Part print with two shaded views. Sizes in mm from the minimum x, y, z corner. Give positions to 0.01 mm unless a question says otherwise; leave off trailing zeros. Write each loop counter-clockwise with the first axis right and the second up, starting at its lowest first coordinate (ties: lowest second). Pieces come first, ordered by that corner, then holes. Notation, with made-up numbers: (-1.75, 65.25) - (29.25, 65.25) arc R32 cw to (29.25, 96.25) - close; hole circle Ø4 at (-13, -25). An arc over 180 degrees is marked (long way). One line per item, written item: value. Start each with the question number.
(1) Probe L1, parallel to Y at x = 3.5, z = 1 (1 decimal); L2, parallel to X at y = 2.5, z = 2.75 (1 decimal); L3, parallel to X at y = 1.25, z = 2.55 (1 decimal). List the from-to ranges inside material, lowest first.
(2) Cut at C-C, the plane y = 4.5. List the corners of the cut face in (x, z) (1 decimal).
(3) Cut at D-D, the plane x = 0.5. List the corners of the cut face in (y, z).
(4) Cut at B-B, the plane z = 0.8. List the corners of the cut face in (x, y).
(5) Mould opens along Y. For the marked faces 1, 2 and 3 say: pulls with the +Y half, pulls with the -Y half, needs draft (parallel to the pull), parting line crosses it, or undercut.
(6) Drop a flat-ended pin along its axis: P1, Ø1.5, axis at x = 9, y = 2, coming from the -Z side. Give the stop position or say it passes through.
(7) Cut at A-A, the plane x = 5.5. List the corners of the cut face in (y, z).
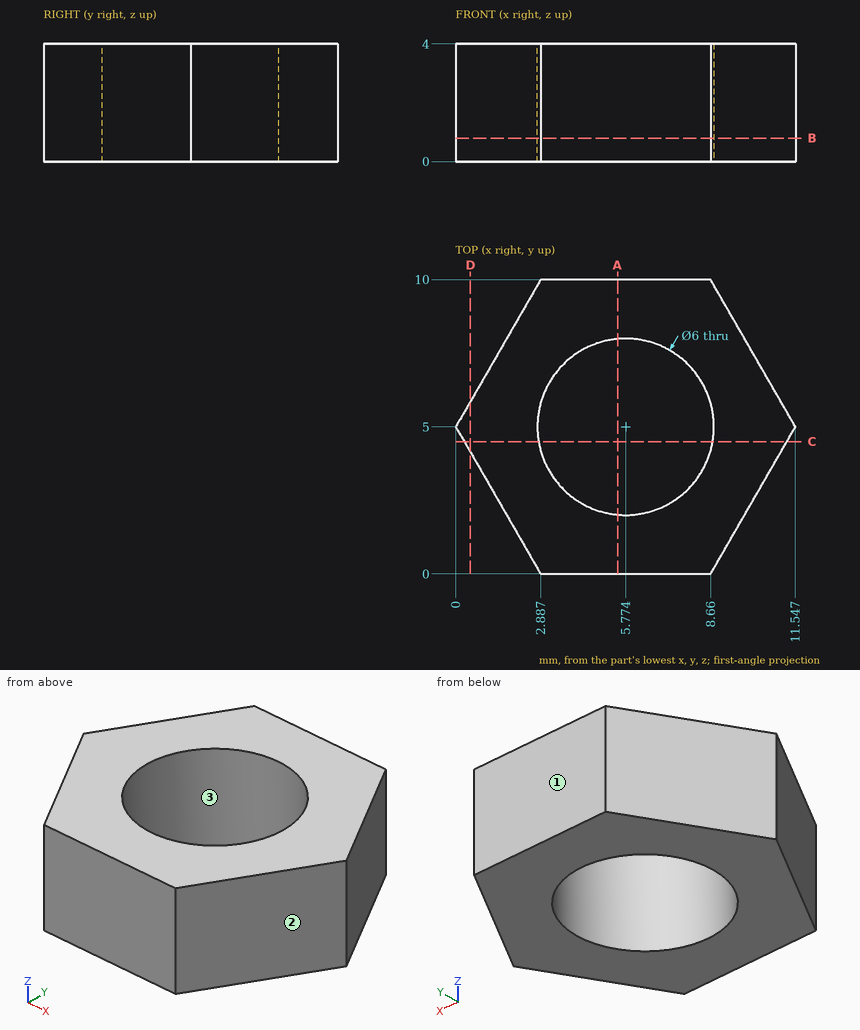
Answers follow:
1. L1: y = 0 to 3, 7 to 10
1. L2: x = 1.4 to 4.1, 7.4 to 10.1
1. L3: x = 2.2 to 9.4
2. outline: (0.3, 0) - (2.8, 0) - (2.8, 4) - (0.3, 4) - close; (8.7, 0) - (11.3, 0) - (11.3, 4) - (8.7, 4) - close
3. outline: (4.13, 0) - (5.87, 0) - (5.87, 4) - (4.13, 4) - close
4. outline: (0, 5) - (2.89, 0) - (8.66, 0) - (11.55, 5) - (8.66, 10) - (2.89, 10) - close; hole circle Ø6 at (5.77, 5)
5. face 1: pulls with the +Y half
5. face 2: pulls with the -Y half
5. face 3: undercut
6. P1: stops at z = 0
7. outline: (0, 0) - (2.01, 0) - (2.01, 4) - (0, 4) - close; (7.99, 0) - (10, 0) - (10, 4) - (7.99, 4) - close
